Geometry check sheet. Reference: the model listing, model coordinates, mm. Round coordinates to 2 decimals unless told otherwise and drop trailing zeros. Order: outer loops, then holes, each group sorted by start corner. A loop starts at its lowest first (then second) coordinate and runs counter-clockwise, first axis right, second up.
(1) Gauge pin test, flat end, axial feed: P1, Ø1.5, axis at x = 1, z = -2, coming from the -Y side. Record the tip position at first contact, or that the pin passes through.
(2) Cross-section at A-A on y = 0. Enter the section's corners in (x, z), and give its area (3 significant figures).
(3) Thickness scan on L1, parallel to Y at x = 0, z = 2; L2, parallel to X at y = -0.1, z = 0.75; L3, parallel to Y at x = -0.5, z = 2.55. Record the ranges inside material, lowest first.
(4) Cross-section at C-C on z = 0.5. Enter the section's corners in (x, y).
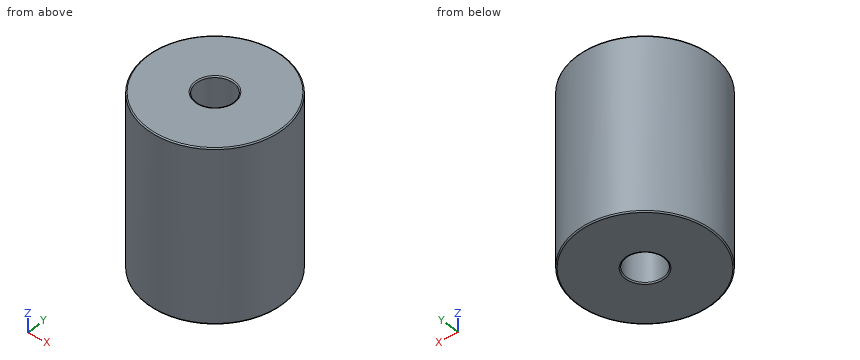
from build123d import *

# Parameters (mm, degrees)
SKETCH3_R                = 2.1828125
SKETCH3_R_2              = 0.5953125
BOSS_EXTRUDE1_DEPTH      = 2.778125
BOSS_EXTRUDE1_DEPTH_BACK = 2.778125
FILLET1_R                = 0.03571875


with BuildPart() as part:
    # Sketch3 → Boss-Extrude1 (new body, two sides)
    with BuildSketch(Plane.XY) as boss_extrude1_sk:
        Circle(SKETCH3_R)
        Circle(SKETCH3_R_2, mode=Mode.SUBTRACT)
    extrude(amount=BOSS_EXTRUDE1_DEPTH)
    extrude(boss_extrude1_sk.sketch, amount=-BOSS_EXTRUDE1_DEPTH_BACK)

    # Fillet1
    fillet1_edges = [part.edges().sort_by_distance(p)[0] for p in [
        (-2.1828125, 0, 2.778125),
        (-0.5953125, 0, 2.778125),
        (-2.1828125, 0, -2.778125),
        (-0.5953125, 0, -2.778125),
    ]]
    fillet(fillet1_edges, radius=FILLET1_R)


solid = part.part
Found:
1. P1: stops at y = -2.17
2. outline: (-2.18, -2.74) arc R0.04 ccw to (-2.15, -2.78) - (-0.63, -2.78) arc R0.04 ccw to (-0.6, -2.74) - (-0.6, 2.74) arc R0.04 ccw to (-0.63, 2.78) - (-2.15, 2.78) arc R0.04 ccw to (-2.18, 2.74) - close; (0.6, -2.74) arc R0.04 ccw to (0.63, -2.78) - (2.15, -2.78) arc R0.04 ccw to (2.18, -2.74) - (2.18, 2.74) arc R0.04 ccw to (2.15, 2.78) - (0.63, 2.78) arc R0.04 ccw to (0.6, 2.74) - close
2. area: 17.6 mm2
3. L1: y = -2.18 to -0.6, 0.6 to 2.18
3. L2: x = -2.18 to -0.59, 0.59 to 2.18
3. L3: y = -2.12 to -0.32, 0.32 to 2.12
4. outline: circle Ø4.37 at (0, 0); hole circle Ø1.19 at (0, 0)
